Verification items for the finished model (mm, model axes). A direction names the side the tool comes from. Give positions to 0.01 mm unless a question says otherwise; leave off trailing zeros. Order: outer loops, then holes, each group sorted by start corner. A loop starts at its lowest first (then second) coordinate and runs counter-clockwise, first axis right, second up.
from build123d import *


with BuildPart() as part:
    # Croquis1 → Revolución1 (revolve)
    with BuildSketch(Plane.XY, mode=Mode.PRIVATE) as revoluci_n1_sk:
        with BuildLine():
            Line((0, 0), (2.5, 0))
            Line((2.5, 0), (2.5, 1.607955914))
            ThreePointArc((2.5, 1.607955914), (2.353553391, 1.961509305), (2, 2.107955914))
            Line((2, 2.107955914), (1.732844387, 2.107955914))
            ThreePointArc((1.732844387, 2.107955914), (1.385515202, 2.248286014), (1.233148974, 2.590506166))
            Line((1.233148974, 2.590506166), (0.370275271, 27.299976083))
            ThreePointArc((0.370275271, 27.299976083), (1.321868208, 29.121568104), (0, 30.695223418))
            Line((0, 30.695223418), (0, 0))
        make_face()
    revolve(revoluci_n1_sk.sketch.rotate(Axis((0, 0, 0), (0, 1, 0)), 90), axis=Axis((0, 0, 0), (0, 1, 0)))


solid = part.part
(1) Set-up check for faces 1 (the flat face through (0, 0, 0)), 2 (the conical face through (-0.24, 15.12, -0.76)): record each of +Z, -Z, +X, -X, +Y, -Y from which the full face is reachable in a straight line by a thin tool's end or side.
Solved:
face 1: +Z, -Z, +X, -X, -Y
face 2: none
(2) Go/stop test with flat-tipped pins: pin 1 (2 mm diameter, centred on x = -1, y = 3.5, fed in from +Z); pin 2 (1 mm diameter, centred on x = -1, y = 19.5, fed in from -Z); pin 3 (1 mm diameter, centred on x = 0, z = 1, fed in from +Y). Record where each tip stops, or that it passes through.
Solved:
pin 1: stops at z = 1.21
pin 2: stops at z = -0.4
pin 3: stops at y = 30.46
(3) Scan lines: line 1 (Y direction, x = -0.05, z = 1.95); line 2 (Y direction, x = 2.35, z = -0.05); line 3 (Z direction, x = -0.85, y = 5.5). Record each from-to range of solid material in increasing order.
Solved:
line 1: y = 0 to 2.11
line 2: y = 0 to 1.96
line 3: z = -0.75 to 0.75
(4) Section check A-A, the plane y = 10.5. Enter the section's corners in (x, z).
Solved:
outline: circle Ø1.91 at (0, 0)
(5) Section check B-B, the plane y = 22. Enter the section's corners in (x, z).
Solved:
outline: circle Ø1.11 at (0, 0)
